Part model, mm, in its own coordinate system. Round coordinates to 2 decimals unless told otherwise and drop trailing zeros. Write each loop counter-clockwise with the first axis right and the second up, starting at its lowest first coordinate (ties: lowest second). Pieces come first, ordered by that corner, then holes.
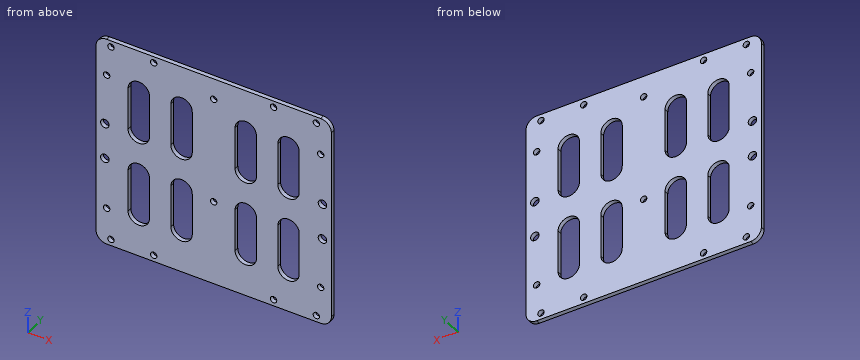
```python
from build123d import *

# Parameters (mm, degrees)
SKETCH_1_W             = 110
SKETCH_1_H             = 100
SKETCH_1_R             = 1.5
SKETCH_1_R_2           = 2
EXTRUDE_1_DEPTH        = 2
FILLET_1_R             = 5
SKETCH_2_R             = 1.5
CUT_EXTRUDE_1129_DEPTH = 10
CUT_EXTRUDE_1751_DEPTH = 10
SKETCH_4_R             = 1.5
CUT_EXTRUDE_1991_DEPTH = 10


with BuildPart() as part:
    # 草图1 → 凸台-拉伸1 (new body)
    with BuildSketch(Plane(origin=(0, 0, 0), x_dir=(1, 0, 0), z_dir=(0, 1, 0))):
        Rectangle(SKETCH_1_W, SKETCH_1_H)
        with Locations(Location((-48, -47, 0), (0, 0, 270))):
            Circle(SKETCH_1_R, mode=Mode.SUBTRACT)
        with Locations(Location((-28, -47, 0), (0, 0, 270))):
            Circle(SKETCH_1_R, mode=Mode.SUBTRACT)
        with Locations(Location((28, -47, 0), (0, 0, 90))):
            Circle(SKETCH_1_R, mode=Mode.SUBTRACT)
        with Locations(Location((48, -47, 0), (0, 0, 90))):
            Circle(SKETCH_1_R, mode=Mode.SUBTRACT)
        with Locations(Location((-50.854561817, 8.5, 0), (0, 0, 270))):
            Circle(SKETCH_1_R_2, mode=Mode.SUBTRACT)
        with Locations(Location((-50.854561817, -8.5, 0), (0, 0, 270))):
            Circle(SKETCH_1_R_2, mode=Mode.SUBTRACT)
        with Locations(Location((50.854561817, -8.5, 0), (0, 0, 90))):
            Circle(SKETCH_1_R_2, mode=Mode.SUBTRACT)
        with Locations(Location((50.854561817, 8.5, 0), (0, 0, 90))):
            Circle(SKETCH_1_R_2, mode=Mode.SUBTRACT)
        with Locations(Location((48, 47, 0), (0, 0, 270))):
            Circle(SKETCH_1_R, mode=Mode.SUBTRACT)
        with Locations(Location((28, 47, 0), (0, 0, 270))):
            Circle(SKETCH_1_R, mode=Mode.SUBTRACT)
        with Locations(Location((-28, 47, 0), (0, 0, 90))):
            Circle(SKETCH_1_R, mode=Mode.SUBTRACT)
        with Locations(Location((-48, 47, 0), (0, 0, 90))):
            Circle(SKETCH_1_R, mode=Mode.SUBTRACT)
    extrude(amount=EXTRUDE_1_DEPTH)

    # 圆角1
    fillet_1_edges = [part.edges().sort_by_distance(p)[0] for p in [
        (55, 1, 50),
        (-55, 1, 50),
        (-55, 1, -50),
        (55, 1, -50),
    ]]
    fillet(fillet_1_edges, radius=FILLET_1_R)

    # 草图2 → Cut-Extrude 1129 (cut)
    with BuildSketch(Plane(origin=(0, 2, 0), x_dir=(1, 0, 0), z_dir=(0, 1, 0))):
        with Locations(Location((0, 10, 0), (0, 0, 270))):
            Circle(SKETCH_2_R)
        with Locations(Location((0, -40, 0), (0, 0, 270))):
            Circle(SKETCH_2_R)
    extrude(amount=-CUT_EXTRUDE_1129_DEPTH, mode=Mode.SUBTRACT)

    # 草图3 → Cut-Extrude 1751 (cut)
    with BuildSketch(Plane.XZ):
        with BuildLine():
            Line((30, -30), (30, -10))
            ThreePointArc((30, -10), (35, -5), (40, -10))
            Line((40, -10), (40, -30))
            ThreePointArc((40, -30), (35, -35), (30, -30))
        make_face()
        with BuildLine():
            Line((10, -30), (10, -10))
            ThreePointArc((10, -10), (15, -5), (20, -10))
            Line((20, -10), (20, -30))
            ThreePointArc((20, -30), (15, -35), (10, -30))
        make_face()
        with BuildLine():
            Line((30, 30), (30, 10))
            ThreePointArc((30, 10), (35, 5), (40, 10))
            Line((40, 10), (40, 30))
            ThreePointArc((40, 30), (35, 35), (30, 30))
        make_face()
        with BuildLine():
            Line((10, 30), (10, 10))
            ThreePointArc((10, 10), (15, 5), (20, 10))
            Line((20, 10), (20, 30))
            ThreePointArc((20, 30), (15, 35), (10, 30))
        make_face()
        with BuildLine():
            Line((-30, -30), (-30, -10))
            ThreePointArc((-30, -10), (-35, -5), (-40, -10))
            Line((-40, -10), (-40, -30))
            ThreePointArc((-40, -30), (-35, -35), (-30, -30))
        make_face()
        with BuildLine():
            Line((-10, -30), (-10, -10))
            ThreePointArc((-10, -10), (-15, -5), (-20, -10))
            Line((-20, -10), (-20, -30))
            ThreePointArc((-20, -30), (-15, -35), (-10, -30))
        make_face()
        with BuildLine():
            Line((-30, 30), (-30, 10))
            ThreePointArc((-30, 10), (-35, 5), (-40, 10))
            Line((-40, 10), (-40, 30))
            ThreePointArc((-40, 30), (-35, 35), (-30, 30))
        make_face()
        with BuildLine():
            Line((-10, 30), (-10, 10))
            ThreePointArc((-10, 10), (-15, 5), (-20, 10))
            Line((-20, 10), (-20, 30))
            ThreePointArc((-20, 30), (-15, 35), (-10, 30))
        make_face()
    extrude(amount=-CUT_EXTRUDE_1751_DEPTH, mode=Mode.SUBTRACT)

    # 草图4 → Cut-Extrude 1991 (cut)
    with BuildSketch(Plane.XZ):
        with Locations(Location((50, 32.5, 0), (0, 0, 270))):
            Circle(SKETCH_4_R)
        with Locations(Location((-50, 32.5, 0), (0, 0, 90))):
            Circle(SKETCH_4_R)
        with Locations(Location((-50, -32.5, 0), (0, 0, 270))):
            Circle(SKETCH_4_R)
        with Locations(Location((50, -32.5, 0), (0, 0, 90))):
            Circle(SKETCH_4_R)
    extrude(amount=-CUT_EXTRUDE_1991_DEPTH, mode=Mode.SUBTRACT)


solid = part.part
```
Q1. Cut at B-B on z = 27. Write the cut outline in (x, y), plus the area to 3 significant figures.
Values follow:
outline: (-55, 0) - (-40, 0) - (-40, 2) - (-55, 2) - close; (-30, 0) - (-20, 0) - (-20, 2) - (-30, 2) - close; (-10, 0) - (10, 0) - (10, 2) - (-10, 2) - close; (20, 0) - (30, 0) - (30, 2) - (20, 2) - close; (40, 0) - (55, 0) - (55, 2) - (40, 2) - close
area: 140 mm2
Q2. Cut at D-D on z = -47. Write the cut outline in (x, y).
Values follow:
outline: (-54.58, 0) - (-49.5, 0) - (-49.5, 2) - (-54.58, 2) - close; (-46.5, 0) - (-29.5, 0) - (-29.5, 2) - (-46.5, 2) - close; (-26.5, 0) - (26.5, 0) - (26.5, 2) - (-26.5, 2) - close; (29.5, 0) - (46.5, 0) - (46.5, 2) - (29.5, 2) - close; (49.5, 0) - (54.58, 0) - (54.58, 2) - (49.5, 2) - close
Q3. Cut at C-C on x = 35. Write the cut outline in (y, z).
Values follow:
outline: (0, -50) - (2, -50) - (2, -35) - (0, -35) - close; (0, -5) - (2, -5) - (2, 5) - (0, 5) - close; (0, 35) - (2, 35) - (2, 50) - (0, 50) - close
Q4. Drop flat-ended pins along their axis: pin 1 (3.5 mm diameter, centred on x = 48, z = 47, fed in from +Y); pin 2 (3.5 mm diameter, centred on x = 50.85, z = 8.5, fed in from -Y). Give the stop position or say it passes through.
Values follow:
pin 1: stops at y = 2
pin 2: passes through
Q5. Cut at A-A on x = 0. Write the cut outline in (y, z), plus the area to 3 significant figures.
Values follow:
outline: (0, -50) - (2, -50) - (2, -11.5) - (0, -11.5) - close; (0, -8.5) - (2, -8.5) - (2, 38.5) - (0, 38.5) - close; (0, 41.5) - (2, 41.5) - (2, 50) - (0, 50) - close
area: 188 mm2
Q6. Wall check: L1, parallel to X at y = 0.2, z = -28.5; L2, parallel to X at y = 1.25, z = 47; L3, parallel to Z at x = -17.5, y = 0.8. Give the ranges that are in metal, low to high.
Values follow:
L1: x = -55 to -40, -30 to -20, -10 to 10, 20 to 30, 40 to 55
L2: x = -54.58 to -49.5, -46.5 to -29.5, -26.5 to 26.5, 29.5 to 46.5, 49.5 to 54.58
L3: z = -50 to -34.33, -5.67 to 5.67, 34.33 to 50
